The model under review builds one solid part; all positions refer to its coordinate system, in mm. Face numbers are marked on the shaded views. A direction names the side the tool comes from. Round coordinates to 2 decimals unless told otherwise and drop trailing zeros. Loops run counter-clockwise (first coordinate to the right, second up) from the corner with the lowest first, then second, coordinate; pieces in that order, holes last. Notation, with made-up numbers: (-1.5, 37) -> (8.5, 37) arc R31 ccw to (8.5, 66) -> close; hole circle Ø2 at (63, 34.25). An arc over 180 degrees is marked (long way). Write each question's results on one line, items separated by ' | '. Start each with the question number.
Item 1: We need section C-C (z = 2.25). Give the boundary of the cut face in (x, y), and give its area (3 significant figures).
Item 2: We need section A-A (y = 17.75). Give the boundary of the cut face in (x, z).
Item 3: We need section D-D (y = 23). Give the boundary of the cut face in (x, z).
Item 4: Tool access review of the marked faces 1, 2 and 3: name each direction out of +Z, -Z, +X, -X, +Y, -Y from which nothing blocks a thin tool from reaching the whole face with its end or side.
Item 5: We need section B-B (x = 18). Give the boundary of the cut face in (y, z), and give its area (3 significant figures).
Item 6: For L1, parallel to X at y = 17.5, z = 7.25; L2, parallel to Y at x = 32.5, z = 4; L3, parallel to Y at x = 5, z = 11.5, list the stretches that pass through material, from the lowest coordinate up. Write a range as from..to.
Item 7: Mouldability with a two-part tool opening along Y and no side actions: class the marked faces 4, 5, 6 and 7 as pulls with the +Y half, pulls with the -Y half, needs draft (parallel to the pull), parting line crosses it, or undercut.
Item 8: Clearance check with flat-ended pins moving along their axes: pin 1 Ø6.5 at (x, y) = (16.5, 8.5) entering from -Z; pin 2 Ø0.8 at (x, z) = (1.5, 12.5) entering from -Y; pin 3 Ø5 at (x, y) = (2, 10) entering from +Z; pin 4 Ø2 at (x, y) = (33, 9.5) entering from +Z. State where each tip first meets the part, or that it passes through.
from build123d import *

# Parameters (mm, degrees)
SKETCH_1_W          = 35
SKETCH_1_H          = 26
SKETCH_1_R          = 1.25
EXTRUDE_1_DEPTH     = 15
CUT_EXTRUDE_1_DEPTH = 7.5
FILLET_1_R          = 1.5
FILLET_2_R          = 0.5
CUT_EXTRUDE_START   = -10
SKETCH_8_R          = 1.5
CUT_EXTRUDE_5_DEPTH = 10
CUT_EXTRUDE_6_DEPTH = 7.5
FILLET_3_R          = 2
SKETCH_10_R         = 4
CUT_EXTRUDE_7_DEPTH = 7.5


with BuildPart() as part:
    # Эскиз1 → Вытянуть1 (new body)
    with BuildSketch(Plane.XY):
        with Locations((17.5, 13)):
            Rectangle(SKETCH_1_W, SKETCH_1_H)
        with Locations((2.5, 9.5)):
            Circle(SKETCH_1_R, mode=Mode.SUBTRACT)
        with Locations((32.5, 9.5)):
            Circle(SKETCH_1_R, mode=Mode.SUBTRACT)
    extrude(amount=EXTRUDE_1_DEPTH)

    # Эскиз2 → Вырез-Вытянуть1 (cut)
    with BuildSketch(Plane(origin=(0, 0, 0), x_dir=(-1, 0, 0), z_dir=(0, 0, -1))):
        with BuildLine():
            Line((-30, 2), (-5, 2))
            Line((-5, 2), (-5, 16.25))
            ThreePointArc((-5, 16.25), (-3.5, 17.75), (-5, 19.25))
            Line((-5, 19.25), (-5, 24))
            Line((-5, 24), (-30, 24))
            Line((-30, 24), (-30, 19.25))
            ThreePointArc((-30, 19.25), (-31.5, 17.75), (-30, 16.25))
            Line((-30, 16.25), (-30, 2))
        make_face()
    extrude(amount=-CUT_EXTRUDE_1_DEPTH, mode=Mode.SUBTRACT)

    # Скругление1
    fillet_1_edges = [part.edges().sort_by_distance(p)[0] for p in [
        (30, 24, 3.75),
        (5, 24, 3.75),
        (5, 2, 3.75),
        (30, 2, 3.75),
    ]]
    fillet(fillet_1_edges, radius=FILLET_1_R)

    # Скругление2
    fillet_2_edges = [part.edges().sort_by_distance(p)[0] for p in [
        (17.5, 0, 15),
        (0, 13, 15),
        (35, 13, 15),
        (17.5, 26, 15),
    ]]
    fillet(fillet_2_edges, radius=FILLET_2_R)

    # Эскиз8 → Вырез-Вытянуть5 (cut)
    with BuildSketch(Plane.XY.offset(15).offset(CUT_EXTRUDE_START)):
        with Locations(Location((5, 17.75, 0), (0, 0, 180))):
            Circle(SKETCH_8_R)
        with Locations(Location((30, 17.75, 0), (0, 0, 180))):
            Circle(SKETCH_8_R)
        with BuildLine():
            Line((9.35, 11.5), (25.65, 11.5))
            ThreePointArc((25.65, 11.5), (26.710660172, 11.939339828), (27.15, 13))
            Line((27.15, 13), (27.15, 22.5))
            ThreePointArc((27.15, 22.5), (26.710660172, 23.560660172), (25.65, 24))
            Line((25.65, 24), (9.35, 24))
            ThreePointArc((9.35, 24), (8.289339828, 23.560660172), (7.85, 22.5))
            Line((7.85, 22.5), (7.85, 13))
            ThreePointArc((7.85, 13), (8.289339828, 11.939339828), (9.35, 11.5))
        make_face()
    extrude(amount=CUT_EXTRUDE_5_DEPTH, mode=Mode.SUBTRACT)

    # Эскиз9 → Вырез-Вытянуть6 (cut)
    with BuildSketch(Plane.XY.offset(15)):
        with BuildLine():
            Line((2.5, 7.25), (-1.280678269, 7.25))
            Line((-1.280678269, 7.25), (-1.280678269, 11.75))
            Line((-1.280678269, 11.75), (2.5, 11.75))
            ThreePointArc((2.5, 11.75), (4.75, 9.5), (2.5, 7.25))
        make_face()
        with BuildLine():
            Line((32.5, 7.25), (36.280678269, 7.25))
            Line((36.280678269, 7.25), (36.280678269, 11.75))
            Line((36.280678269, 11.75), (32.5, 11.75))
            ThreePointArc((32.5, 11.75), (30.25, 9.5), (32.5, 7.25))
        make_face()
    extrude(amount=-CUT_EXTRUDE_6_DEPTH, mode=Mode.SUBTRACT)

    # Скругление3
    # the kernel refuses this fillet: 2 mm, written as the material it takes off along each edge
    with BuildSketch(Plane(origin=(33, 24, 15), x_dir=(1, 0, 0), z_dir=(0, -1, 0))) as fillet_3_piece_1:
        with BuildLine():
            CenterArc((1.5, -0.5), 0.5, 0, 90)
            Line((2, -0.5), (2, 0))
            Line((2, 0), (1.5, 0))
        make_face()
    revolve(axis=Axis((33, 24, 15), (0, 0, 1)), revolution_arc=90, mode=Mode.SUBTRACT)
    with BuildSketch(Plane(origin=(2, 24, 15), x_dir=(0, 1, 0), z_dir=(1, 0, 0))) as fillet_3_piece_2:
        with BuildLine():
            CenterArc((1.5, -0.5), 0.5, 0, 90)
            Line((2, -0.5), (2, 0))
            Line((2, 0), (1.5, 0))
        make_face()
    revolve(axis=Axis((2, 24, 15), (0, 0, 1)), revolution_arc=90, mode=Mode.SUBTRACT)
    with BuildSketch(Plane(origin=(33, 2, 15), x_dir=(0, -1, 0), z_dir=(-1, 0, 0))) as fillet_3_piece_3:
        with BuildLine():
            CenterArc((1.5, -0.5), 0.5, 0, 90)
            Line((2, -0.5), (2, 0))
            Line((2, 0), (1.5, 0))
        make_face()
    revolve(axis=Axis((33, 2, 15), (0, 0, 1)), revolution_arc=90, mode=Mode.SUBTRACT)
    with BuildSketch(Plane(origin=(2, 2, 15), x_dir=(-1, 0, 0), z_dir=(0, 1, 0))) as fillet_3_piece_4:
        with BuildLine():
            CenterArc((1.5, -0.5), 0.5, 0, 90)
            Line((2, -0.5), (2, 0))
            Line((2, 0), (1.5, 0))
        make_face()
    revolve(axis=Axis((2, 2, 15), (0, 0, 1)), revolution_arc=90, mode=Mode.SUBTRACT)
    with BuildSketch(Plane(origin=(0, 0, -5), x_dir=(1, 0, 0), z_dir=(0, 0, 1)), Plane(origin=(0, 26, -5), x_dir=(0, -1, 0), z_dir=(0, 0, 1))) as fillet_3_piece_5:
        with BuildLine():
            CenterArc((FILLET_3_R, FILLET_3_R), FILLET_3_R, 180, 90)
            Line((0, FILLET_3_R), (0, 0))
            Line((0, 0), (FILLET_3_R, 0))
        make_face()
    extrude(amount=20, mode=Mode.SUBTRACT)
    with BuildSketch(Plane(origin=(35, 0, -5), x_dir=(-1, 0, 0), z_dir=(0, 0, 1)), Plane(origin=(35, 26, -5), x_dir=(0, -1, 0), z_dir=(0, 0, 1))) as fillet_3_piece_6:
        with BuildLine():
            CenterArc((FILLET_3_R, -FILLET_3_R), FILLET_3_R, 90, 90)
            Line((0, -FILLET_3_R), (0, 0))
            Line((0, 0), (FILLET_3_R, 0))
        make_face()
    extrude(amount=20, mode=Mode.SUBTRACT)

    # Эскиз10 → Вырез-Вытянуть7 (cut)
    with BuildSketch(Plane(origin=(0, 0, 0), x_dir=(-1, 0, 0), z_dir=(0, 0, -1))):
        with Locations((-5, 17.75)):
            Circle(SKETCH_10_R)
        with Locations((-30, 17.75)):
            Circle(SKETCH_10_R)
    extrude(amount=-CUT_EXTRUDE_7_DEPTH, mode=Mode.SUBTRACT)


solid = part.part
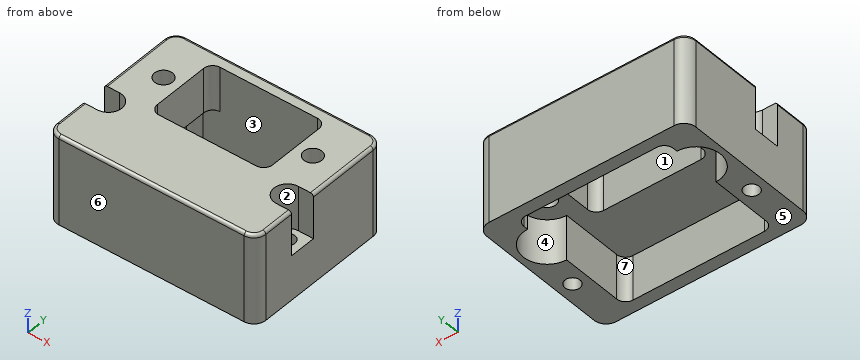
Here are the results:
1) outline: (0, 2) arc R2 ccw to (2, 0) -> (33, 0) arc R2 ccw to (35, 2) -> (35, 24) arc R2 ccw to (33, 26) -> (2, 26) arc R2 ccw to (0, 24) -> close; hole circle Ø2.5 at (2.5, 9.5); hole (5, 3.5) arc R1.5 ccw to (6.5, 2) -> (28.5, 2) arc R1.5 ccw to (30, 3.5) -> (30, 13.75) arc R4 ccw to (30, 21.75) -> (30, 22.5) arc R1.5 ccw to (28.5, 24) -> (6.5, 24) arc R1.5 ccw to (5, 22.5) -> (5, 21.75) arc R4 ccw to (5, 13.75) -> close; hole circle Ø2.5 at (32.5, 9.5) | area: 298 mm2
2) outline: (0, 0) -> (1, 0) -> (1, 7.5) -> (3.5, 7.5) -> (3.5, 15) -> (0.5, 15) arc R0.5 ccw to (0, 14.5) -> close; (6.5, 7.5) -> (7.85, 7.5) -> (7.85, 15) -> (6.5, 15) -> close; (27.15, 7.5) -> (28.5, 7.5) -> (28.5, 15) -> (27.15, 15) -> close; (31.5, 7.5) -> (34, 7.5) -> (34, 0) -> (35, 0) -> (35, 14.5) arc R0.5 ccw to (34.5, 15) -> (31.5, 15) -> close
3) outline: (0, 0) -> (5.09, 0) -> (5.09, 7.5) -> (7.94, 7.5) -> (7.94, 15) -> (0.5, 15) arc R0.5 ccw to (0, 14.5) -> close; (27.06, 7.5) -> (29.91, 7.5) -> (29.91, 0) -> (35, 0) -> (35, 14.5) arc R0.5 ccw to (34.5, 15) -> (27.06, 15) -> close
4) face 1: +Z, -Z | face 2: +Z, +X | face 3: -Z
5) outline: (0, 0) -> (2, 0) -> (2, 7.5) -> (11.5, 7.5) -> (11.5, 15) -> (0.5, 15) arc R0.5 ccw to (0, 14.5) -> close; (24, 0) -> (26, 0) -> (26, 14.5) arc R0.5 ccw to (25.5, 15) -> (24, 15) -> close | area: 131 mm2
6) L1: x = 0..1.01, 33.99..35 | L2: y = 0..8.25, 10.75..14.63, 20.87..26 | L3: y = 0..16.25, 19.25..26
7) face 4: undercut | face 5: needs draft | face 6: pulls with the -Y half | face 7: undercut
8) pin 1: stops at z = 7.5 | pin 2: stops at y = 0 | pin 3: stops at z = 15 | pin 4: stops at z = 7.5
